The figure shows three views and two pictorial views of one solid part (mm, origin at its lowest corner). Answer the questions. Round coordinates to 2 decimals unless told otherwise and drop trailing zeros. Order: outer loops, then holes, each group sorted by start corner. A loop starts at its lowest first (then second) coordinate and runs counter-clockwise, first axis right, second up. Notation, with made-up numbers: (-27.5, 58.25) -> (25.5, 58.25) arc R17 ccw to (25.5, 91.25) -> close; hole circle Ø3 at (40, 58). An arc over 180 degrees is marked (long way). Answer in a Markdown table with one row per item. Add a question column.
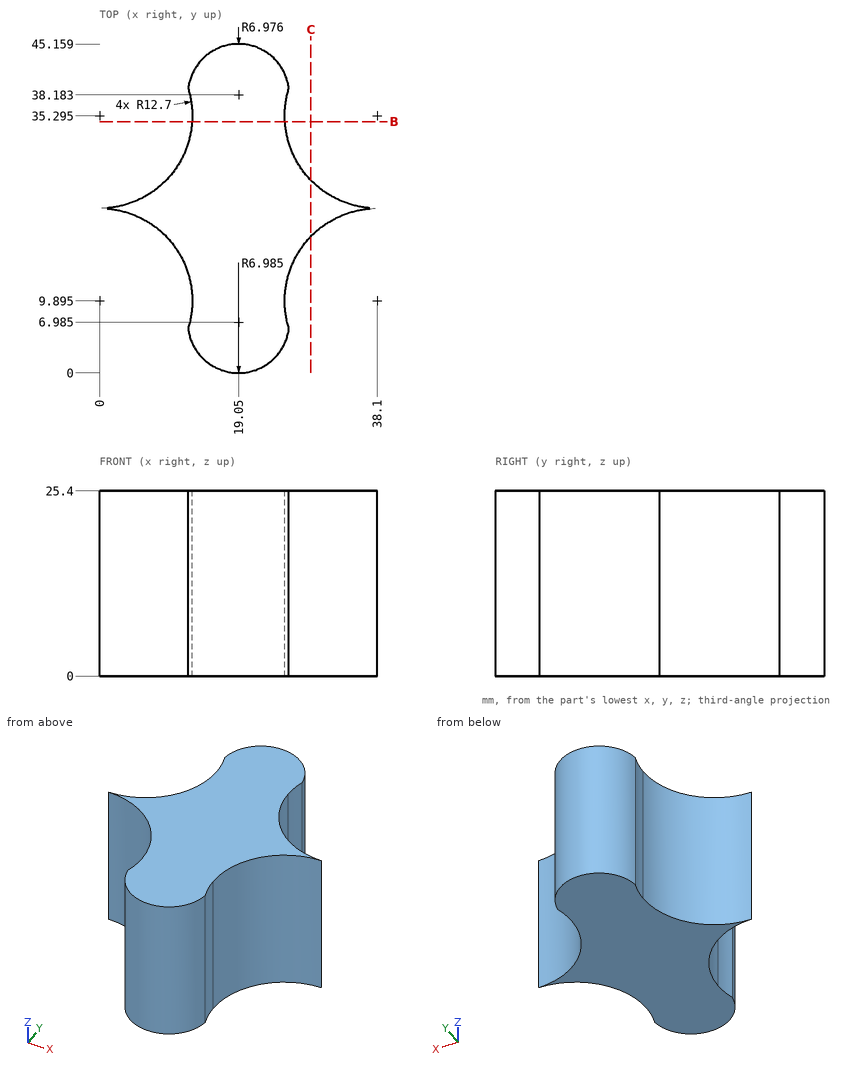
1. Each of these flat-tipped pins is pushed along its axis until it touches: pin 1 (8 mm diameter, centred on x = 31, z = 7, fed in from -Y); pin 2 (1 mm diameter, centred on y = 8, z = 4, fed in from -X); pin 3 (5 mm diameter, centred on y = 30, z = 4, fed in from -X). Where does it stop, or does it pass through?
2. Straight lines are drawn through the part: line 1 along Y through (x, z) = (13, 11.75); line 2 along X through (y, z) = (14, 3.25); line 3 along Y through (x, z) = (34.5, 12.5). For each, find the intervals that lie inside material, in ascending order.
3. The part is cut by section B-B (y = 34.5). Give the vertices of the cut face in (x, z) (3 decimals), then the cut area to 3 significant figures.
4. The part is cut by section C-C (x = 29). Give the vertices of the cut face in (y, z), then the cut area to 3 significant figures.
Report:
| question | item | result |
|---|---|---|
| 1 | pin 1 | stops at y = 16.07 |
| 1 | pin 2 | stops at x = 12.47 |
| 1 | pin 3 | stops at x = 10.03 |
| 2 | line 1 | y = 3.49 to 41.66 |
| 2 | line 2 | x = 12.02 to 26.08 |
| 2 | line 3 | y = 22.07 to 23.12 |
| 3 | outline | (12.675, 0) -> (25.425, 0) -> (25.425, 25.4) -> (12.675, 25.4) -> close |
| 3 | area | 324 mm^2 |
| 4 | outline | (18.75, 0) -> (26.44, 0) -> (26.44, 25.4) -> (18.75, 25.4) -> close |
| 4 | area | 195 mm^2 |
